The listing builds one solid part. Answer for the finished solid, in the listing's coordinates (mm). A direction names the side the tool comes from. Round coordinates to 2 decimals unless told otherwise and drop trailing zeros. Write each loop counter-clockwise with the first axis right and the second up, starting at its lowest first coordinate (ties: lowest second). Pieces come first, ordered by that corner, then holes. Notation, with made-up numbers: (28.5, 35.25) - (40.5, 35.25) arc R25 cw to (40.5, 64.25) - close; hole circle Ø9 at (34, -0.5). An arc over 180 degrees is marked (long way). Return JSON: item names as keys, results as strings. Group by question number.
(1) Section B-B, the plane x = 23 is taken. Write down the section's boundary in (y, z), then the cut area to 3 significant figures.
(2) Section D-D, the plane z = 15 is taken. Write down the section's boundary in (x, y), then the cut area to 3 significant figures.
(3) Section A-A, the plane z = -6.5 is taken. Write down the section's boundary in (x, y), then the cut area to 3 significant figures.
(4) Section C-C, the plane y = -39 is taken. Write down the section's boundary in (x, z).
(5) Find the intervals of material crossed by line 1 along X through (y, z) = (4, 30); line 2 along Y through (x, z) = (-6, 37); line 3 along Y through (x, z) = (-12, -35.5), in increasing order. Write a range as [from, to].
(6) Determine the mould class of faces 1 (the flat face through (1, 5, -52)), 2 (the flat face through (-49, 5, 1)), 3 (the flat face through (-52, 5, -1)) for opening direction Z: +Z half, -Z half, draft (parallel to the pull), parting line (faces both ways), or undercut.
(7) Which of the six approach directions +Z, -Z, +X, -X, +Y, -Y give full straight-line access (tool end or side, diameter ignored) to faces 4 (the flat face through (41.306, -25.193, -19.706)), 5 (the cylindrical face through (-27.98, -4.93, 27.88)), 6 (the flat face through (-0.728, -87.281, -41.508)), 7 (the flat face through (-18, -102, -18)), 8 (the flat face through (0, -51.9, 29.7))?
(8) Each of these flat-tipped pins is pushed along its axis until it touches: pin 1 (13.5 mm diameter, centred on x = 31.5, z = -35, fed in from +Y); pin 2 (1.5 mm diameter, centred on x = -4.5, y = -92, fed in from -Z); pin 3 (5 mm diameter, centred on x = -37.5, y = -32.5, fed in from +Z). Where does it stop, or does it pass through?
```python
from build123d import *

# Parameters (mm, degrees)
ESQUISSE1_W                  = 104
ESQUISSE1_H                  = 104
BOSS_EXTRU_2_DEPTH           = 56
BOSS_EXTRU_2_DRAFT           = -23
SYM_TRIE1_COPY_1_SKETCH_W    = 104
SYM_TRIE1_COPY_1_SKETCH_H    = 104
SYM_TRIE1_COPY_1_DEPTH       = 56
SYM_TRIE1_COPY_1_DRAFT       = -23
ENL_V_MAT_EXTRU_1_DEPTH      = 134.985073796
ENL_V_MAT_EXTRU_1_DEPTH_BACK = 134.985073796
ESQUISSE2_R                  = 25
CONG_1_R                     = 15
ESQUISSE3_W                  = 52
ESQUISSE3_H                  = 52
ENL_V_MAT_EXTRU_2_DEPTH      = 134.985073796
ESQUISSE4_R                  = 35
ENL_V_MAT_EXTRU_3_DEPTH      = 10
BOSS_EXTRU_3_DEPTH           = 10
CONG_2_R                     = 5
ENL_V_MAT_EXTRU_4_DEPTH      = 10


with BuildPart() as part:
    # Esquisse1 → Boss.-Extru.2 (with draft: the straight prism first)
    with BuildSketch(Plane(origin=(0, 0, 0), x_dir=(1, 0, 0), z_dir=(0, 1, 0))):
        Rectangle(ESQUISSE1_W, ESQUISSE1_H)
    extrude(amount=-BOSS_EXTRU_2_DEPTH)
    # Boss.-Extru.2: the draft: its side faces are tilted about the plane it starts from
    boss_extru_2_sides = [part.faces().sort_by_distance(p)[0] for p in [
        (-52, -28, 0),
        (0, -28, 52),
        (52, -28, 0),
        (0, -28, -52),
    ]]
    draft(boss_extru_2_sides, Plane(origin=(0, 0, 0), x_dir=(1, 0, 0), z_dir=(0, 1, 0)), BOSS_EXTRU_2_DRAFT)


with BuildPart() as sym_trie1_copy_1_tool:
    # Symétrie1 copy 1 sketch → Symétrie1 copy 1 (with draft: the straight prism first)
    with BuildSketch(Plane.XZ.offset(112)):
        Rectangle(SYM_TRIE1_COPY_1_SKETCH_W, SYM_TRIE1_COPY_1_SKETCH_H)
    extrude(amount=-SYM_TRIE1_COPY_1_DEPTH)
    # Symétrie1 copy 1: the draft: its side faces are tilted about the plane it starts from
    sym_trie1_copy_1_sides = [sym_trie1_copy_1_tool.faces().sort_by_distance(p)[0] for p in [
        (-52, -84, 0),
        (0, -84, 52),
        (52, -84, 0),
        (0, -84, -52),
    ]]
    draft(sym_trie1_copy_1_sides, Plane.XZ.offset(112), SYM_TRIE1_COPY_1_DRAFT)


with BuildPart() as part_1:
    add(part.part)

    # Symétrie1 copy 1: add sym_trie1_copy_1_tool
    add(sym_trie1_copy_1_tool.part)

    # Esquisse2 → Enlèv. mat.-Extru.1 (cut, two sides: drawn at the far end of the back side and taken through both)
    with BuildSketch(Plane(origin=(0, 0, 0), x_dir=(1, 0, 0), z_dir=(0, 1, 0)).offset(-ENL_V_MAT_EXTRU_1_DEPTH_BACK)):
        with Locations(Location((0, 0, 0), (0, 0, 270))):
            Circle(ESQUISSE2_R)
    extrude(amount=ENL_V_MAT_EXTRU_1_DEPTH + ENL_V_MAT_EXTRU_1_DEPTH_BACK, mode=Mode.SUBTRACT)

    # Congé1
    cong_1_edges = [part_1.edges().sort_by_distance(p)[0] for p in [
        (-28.229410292, -56, 0),
        (0, -56, 28.229410292),
        (28.229410292, -56, 0),
        (0, -56, -28.229410292),
    ]]
    fillet(cong_1_edges, radius=CONG_1_R)

    # Esquisse3 → Enlèv. mat.-Extru.2 (cut, through all)
    with BuildSketch(Plane(origin=(0, 0, 0), x_dir=(1, 0, 0), z_dir=(0, 1, 0))):
        with Locations((26, -26)):
            Rectangle(ESQUISSE3_W, ESQUISSE3_H)
    extrude(amount=-ENL_V_MAT_EXTRU_2_DEPTH, mode=Mode.SUBTRACT)

    # Esquisse4 → Enlèv. mat.-Extru.3 (cut)
    with BuildSketch(Plane(origin=(0, 0, 0), x_dir=(1, 0, 0), z_dir=(0, 1, 0))):
        Circle(ESQUISSE4_R)
    enl_v_mat_extru_3 = extrude(amount=-ENL_V_MAT_EXTRU_3_DEPTH, mode=Mode.SUBTRACT)

    # Symétrie2: Enlèv. mat.-Extru.3 across plane
    add(enl_v_mat_extru_3.mirror(Plane.ZX.offset(-56)), mode=Mode.SUBTRACT)

    # Esquisse7 → Boss.-Extru.3 (add)
    with BuildSketch(Plane(origin=(0, 0, 0), x_dir=(1, 0, 0), z_dir=(0, 1, 0))):
        Polygon((-52, -52), (0, -52), (0, -49), (-49, -49), (-49, 49), (49, 49), (49, 0), (52, 0), (52, 52), (-52, 52), align=None)
    extrude(amount=BOSS_EXTRU_3_DEPTH)

    # Congé2
    cong_2_edges = [part_1.edges().sort_by_distance(p)[0] for p in [
        (-26, 0, 52),
        (-52, 0, 0),
        (0, 0, -52),
        (52, 0, -26),
    ]]
    fillet(cong_2_edges, radius=CONG_2_R)

    # Esquisse8 → Enlèv. mat.-Extru.4 (cut)
    with BuildSketch(Plane(origin=(0, 0, 0), x_dir=(1, 0, 0), z_dir=(0, 1, 0))):
        with BuildLine():
            Line((-38.537319575, 42.779960262), (-27.930717857, 32.173358544))
            ThreePointArc((-27.930717857, 32.173358544), (-27.930717857, 27.930717857), (-32.173358544, 27.930717857))
            Line((-32.173358544, 27.930717857), (-42.779960262, 38.537319575))
            ThreePointArc((-42.779960262, 38.537319575), (-42.779960262, 42.779960262), (-38.537319575, 42.779960262))
        make_face()
        with BuildLine():
            Line((42.779960262, 38.537319575), (32.173358544, 27.930717857))
            ThreePointArc((32.173358544, 27.930717857), (27.930717857, 27.930717857), (27.930717857, 32.173358544))
            Line((27.930717857, 32.173358544), (38.537319575, 42.779960262))
            ThreePointArc((38.537319575, 42.779960262), (42.779960262, 42.779960262), (42.779960262, 38.537319575))
        make_face()
        with BuildLine():
            Line((38.537319575, -42.779960262), (27.930717857, -32.173358544))
            ThreePointArc((27.930717857, -32.173358544), (27.930717857, -27.930717857), (32.173358544, -27.930717857))
            Line((32.173358544, -27.930717857), (42.779960262, -38.537319575))
            ThreePointArc((42.779960262, -38.537319575), (42.779960262, -42.779960262), (38.537319575, -42.779960262))
        make_face()
        with BuildLine():
            Line((-42.779960262, -38.537319575), (-32.173358544, -27.930717857))
            ThreePointArc((-32.173358544, -27.930717857), (-27.930717857, -27.930717857), (-27.930717857, -32.173358544))
            Line((-27.930717857, -32.173358544), (-38.537319575, -42.779960262))
            ThreePointArc((-38.537319575, -42.779960262), (-42.779960262, -42.779960262), (-42.779960262, -38.537319575))
        make_face()
    extrude(amount=-ENL_V_MAT_EXTRU_4_DEPTH, mode=Mode.SUBTRACT)


solid = part_1.part
```
Working result:
{
 "1": {"outline": "(-112, -52) - (-61.86, -30.72) arc R15 cw to (-50.14, -30.72) - (-0.94, -51.6) arc R5 ccw to (1.02, -52) - (10, -52) - (10, -49) - (0, -49) - (0, -26.38) - (-10, -26.38) - (-10, -9.8) - (-102, -9.8) - (-102, -26.38) - (-112, -26.38) - close", "area": "3,100 mm^2"},
 "2": {"outline": "(-52, -112) - (-31.62, -112) - (-31.62, -102) - (-20, -102) - (-20, -10) - (-31.62, -10) - (-31.62, 0) - (-49, 0) - (-49, 10) - (-52, 10) - (-52, 1.02) arc R5 ccw to (-51.6, -0.94) - (-30.72, -50.14) arc R15 cw to (-30.72, -61.86) - close", "area": "2,060 mm^2"},
 "3": {"outline": "(-52, -112) - (-34.39, -112) - (-34.39, -102) - (-24.14, -102) - (-24.14, -10) - (-34.39, -10) - (-34.39, 0) - (-49, 0) - (-49, 10) - (-52, 10) - (-52, 1.02) arc R5 ccw to (-51.6, -0.94) - (-30.72, -50.14) arc R15 cw to (-30.72, -61.86) - close; (24.14, -102) - (34.39, -102) - (34.39, -112) - (52, -112) - (30.72, -61.86) arc R15 cw to (30.72, -50.14) - (51.6, -0.94) arc R5 ccw to (52, 1.02) - (52, 10) - (49, 10) - (49, 0) - (34.39, 0) - (34.39, -10) - (24.14, -10) - close", "area": "3,240 mm^2"},
 "4": {"outline": "(-35.45, -35.45) - (35.45, -35.45) - (35.45, 0) - (25, 0) arc R25 cw (long way) to (0, 25) - (0, 35.45) - (-35.45, 35.45) - close"},
 "5": {"line 1": "x = [-52, -49]", "line 2": "y = [-112, -76.66], [-35.34, 0]", "line 3": "y = [-112, -73.13], [-38.87, 0]"},
 "6": {"face 1": "-Z half", "face 2": "undercut", "face 3": "draft"},
 "7": {"face 4": "+Z, -Z, +X", "face 5": "+Y", "face 6": "-Z, +X, -X", "face 7": "-Y", "face 8": "+Z, +X, +Y, -Y"},
 "8": {"pin 1": "stops at y = 0", "pin 2": "stops at z = -43.83", "pin 3": "stops at z = 39.27"}
}
